from build123d import *

# Parameters (mm, degrees)
SKETCH_1_R      = 17.5
SKETCH_1_R_2    = 4
EXTRUDE_1_DEPTH = 9.25
FILLET_1_R      = 2.5
FILLET_2_R      = 0.5


with BuildPart() as part:
    # 草图1 → 凸台-拉伸1 (new, symmetric)
    with BuildSketch(Plane.XY):
        Circle(SKETCH_1_R)
        Circle(SKETCH_1_R_2, mode=Mode.SUBTRACT)
    extrude(amount=EXTRUDE_1_DEPTH, both=True)

    # 圆角1
    fillet_1_edges = [part.edges().sort_by_distance(p)[0] for p in [
        (-17.5, 0, -9.25),
        (-17.5, 0, 9.25),
    ]]
    fillet(fillet_1_edges, radius=FILLET_1_R)

    # 圆角2
    fillet_2_edges = [part.edges().sort_by_distance(p)[0] for p in [
        (-4, 0, -9.25),
        (-4, 0, 9.25),
    ]]
    fillet(fillet_2_edges, radius=FILLET_2_R)


solid = part.part
CAD build for the part. Positions are in the model's coordinates, mm. Coordinates: 2 decimals unless noted, no trailing zeros. Loops run counter-clockwise (first coordinate to the right, second up) from the corner with the lowest first, then second, coordinate; pieces in that order, holes last. Notation, with made-up numbers: (18.25, 46.25) -> (41.25, 46.25) arc R20 ccw to (41.25, 78.25) -> close; hole circle Ø3 at (26, 64.25). An arc over 180 degrees is marked (long way). One line per item, written item: value.
1. Slice it at A-A on x = 0. Write the cut outline in (y, z), and give its area (3 significant figures).
Answers:
outline: (-17.5, -6.75) arc R2.5 ccw to (-15, -9.25) -> (-4.5, -9.25) arc R0.5 ccw to (-4, -8.75) -> (-4, 8.75) arc R0.5 ccw to (-4.5, 9.25) -> (-15, 9.25) arc R2.5 ccw to (-17.5, 6.75) -> close; (4, -8.75) arc R0.5 ccw to (4.5, -9.25) -> (15, -9.25) arc R2.5 ccw to (17.5, -6.75) -> (17.5, 6.75) arc R2.5 ccw to (15, 9.25) -> (4.5, 9.25) arc R0.5 ccw to (4, 8.75) -> close
area: 494 mm^2
2. Pull direction Y, two halves, no side cores. Call faces 1 (the face through (-0.867, -3.905, -0.123)), 2 (the face through (3, 4, 9.25)), 3 (the face through (-13.887, -10.648, 0.095)): pulls with the +Y half, pulls with the -Y half, needs draft (parallel to the pull), parting line crosses it, or undercut.
Answers:
face 1: undercut
face 2: needs draft
face 3: parting line crosses it
3. Flat gauge pins, fed straight in: P1, Ø1, axis at y = -5, z = 3, coming from the -X side; P2, Ø4, axis at x = -5.5, z = 0, coming from the +Y side; P3, Ø3, axis at x = 11, z = -3.5, coming from the +Y side. Where does each tip first touch, or does it go through?
Answers:
P1: stops at x = -16.91
P2: stops at y = 17.15
P3: stops at y = 14.7
4. Drill centre lines: line 1 (Y direction, x = 0, z = -2); line 2 (X direction, y = 1.5, z = 5.25); line 3 (X direction, y = 9.5, z = -7.25). Where is each one in solid material? Low to high. Write a range as [from, to].
Answers:
line 1: y = [-17.5, -4], [4, 17.5]
line 2: x = [-17.44, -3.71], [3.71, 17.44]
line 3: x = [-14.64, 14.64]
5. Slice it at C-C on z = 3. Write the cut outline in (x, y), and give its area (3 significant figures).
Answers:
outline: circle Ø35 at (0, 0); hole circle Ø8 at (0, 0)
area: 912 mm^2
